Could you check a few things on this drawing? It's one solid part, dimensions in mm from its lowest x, y, z. Round coordinates to 2 decimals unless told otherwise and drop trailing zeros. Write each loop counter-clockwise with the first axis right and the second up, starting at its lowest first coordinate (ties: lowest second). Pieces come first, ordered by that corner, then holes. Notation, with made-up numbers: (27, 11) - (60, 11) arc R20 ccw to (60, 39) - close; hole circle Ø5 at (-10, 27.25). An arc over 180 degrees is marked (long way). Put each result on its own line as item: value.
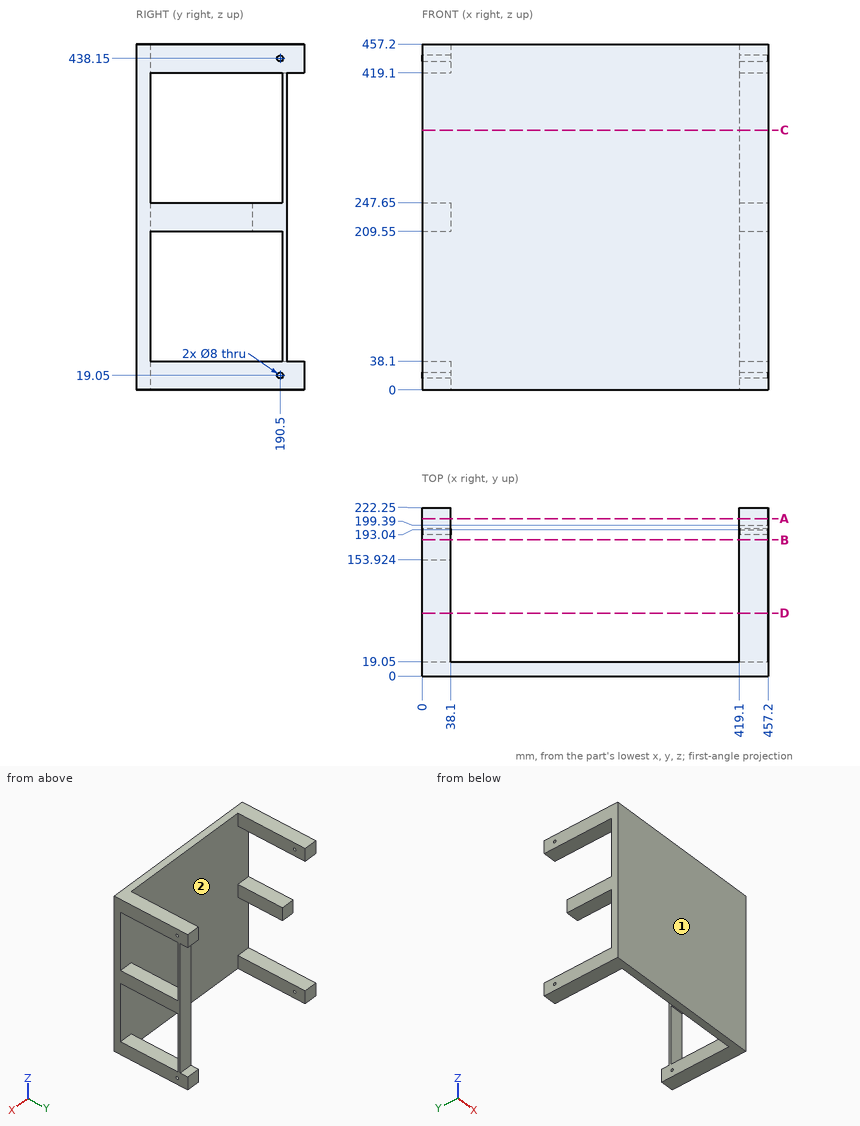
(1) Imagine slicing it at A-A, the plane y = 208. List the corners of the cut face in (x, z) for me, then the cut area to 3 significant figures.
Values found:
outline: (0, 0) - (38.1, 0) - (38.1, 38.1) - (0, 38.1) - close; (0, 419.1) - (38.1, 419.1) - (38.1, 457.2) - (0, 457.2) - close; (419.1, 0) - (457.2, 0) - (457.2, 38.1) - (419.1, 38.1) - close; (419.1, 419.1) - (457.2, 419.1) - (457.2, 457.2) - (419.1, 457.2) - close
area: 5,810 mm^2
(2) Imagine slicing it at C-C, the plane z = 343.5. List the corners of the cut face in (x, y) for me, then the cut area to 3 significant figures.
Values found:
outline: (0, 0) - (457.2, 0) - (457.2, 19.05) - (0, 19.05) - close; (419.1, 193.04) - (457.2, 193.04) - (457.2, 199.39) - (419.1, 199.39) - close
area: 8,950 mm^2
(3) Imagine slicing it at D-D, the plane y = 83. List the corners of the cut face in (x, z) for me, then the cut area to 3 significant figures.
Values found:
outline: (0, 0) - (38.1, 0) - (38.1, 38.1) - (0, 38.1) - close; (0, 209.55) - (38.1, 209.55) - (38.1, 247.65) - (0, 247.65) - close; (0, 419.1) - (38.1, 419.1) - (38.1, 457.2) - (0, 457.2) - close; (419.1, 0) - (457.2, 0) - (457.2, 38.1) - (419.1, 38.1) - close; (419.1, 209.55) - (457.2, 209.55) - (457.2, 247.65) - (419.1, 247.65) - close; (419.1, 419.1) - (457.2, 419.1) - (457.2, 457.2) - (419.1, 457.2) - close
area: 8,710 mm^2
(4) If we mould it in two halves opening along X, with no side actions, what happens to the marked faces 1 and 2? For each: pulls with the +X half, pulls with the -X half, needs draft (parallel to the pull), parting line crosses it, or undercut.
Values found:
face 1: needs draft
face 2: undercut
(5) Please list where these lines run through material, in increasing order: probe 1 along Z at (x, y) = (30, 190); probe 2 along Z at (x, y) = (439, 190); probe 3 along Y at (x, z) = (442.5, 19.05). Write a range as from..to.
Values found:
probe 1: z = 0..15.08, 23.02..38.1, 419.1..434.18, 442.12..457.2
probe 2: z = 0..15.08, 23.02..38.1, 209.55..247.65, 419.1..434.18, 442.12..457.2
probe 3: y = 0..186.5, 194.5..222.25
(6) Imagine slicing it at B-B, the plane y = 180. List the corners of the cut face in (x, z) for me.
Values found:
outline: (0, 0) - (38.1, 0) - (38.1, 38.1) - (0, 38.1) - close; (0, 419.1) - (38.1, 419.1) - (38.1, 457.2) - (0, 457.2) - close; (419.1, 0) - (457.2, 0) - (457.2, 38.1) - (419.1, 38.1) - close; (419.1, 209.55) - (457.2, 209.55) - (457.2, 247.65) - (419.1, 247.65) - close; (419.1, 419.1) - (457.2, 419.1) - (457.2, 457.2) - (419.1, 457.2) - close
(7) I'm going to push flat-ended pins straight in: pin 1 (19 mm diameter, centred on x = 442.5, z = 208, fed in from +Y); pin 2 (6 mm diameter, centred on x = 403.5, z = 281.5, fed in from +Y). Where does each tip first touch, or does it pass through?
Values found:
pin 1: stops at y = 199.39
pin 2: stops at y = 19.05
